Read the model definition and answer for the solid it produces. Units are mm, in the model's axes. A direction names the side the tool comes from. Give positions to 0.01 mm unless a question says otherwise; leave off trailing zeros. Order: outer loops, then holes, each group sorted by start corner. A loop starts at its lowest first (then second) coordinate and runs counter-clockwise, first axis right, second up. Notation, with made-up numbers: (26.25, 17) -> (36.25, 17) arc R4 cw to (36.25, 23) -> close; hole circle Ø11 at (63, 75.25). An arc over 180 degrees is marked (long way). Answer as CSV lines item,"result". Start each with the question number.
1) Find section D-D (x = 0.75). Determine the outline of the cut face in (y, z), and give its area (3 significant figures).
2) For faces 5 (the face through (0, 15, 6)), 6 (the face through (0, 8.019, 7)), 7 (the face through (-12.5, 4, 5)), determine the directions among +Z, -Z, +X, -X, +Y, -Y from which every point of the face is accessible in a straight line to the end or side of a thin tool.
3) Find section B-B (x = -8.5). Determine the outline of the cut face in (y, z).
4) Find section A-A (y = 2.75). Determine the outline of the cut face in (x, z).
5) Flat-ended cylindrical pins translate along their axes: pin 1 Ø5 at (x, z) = (-9, 3) entering from +Y; pin 2 Ø5 at (y, z) = (19, 5.5) entering from +X; pin 3 Ø3.5 at (x, y) = (0, 17) entering from +Z. Find the tip coordinate at first contact, or state that the pin passes through.
6) Straight lines are drawn through the part: L1, parallel to X at y = 3.5, z = 6.75; L2, parallel to X at y = 2.5, z = 6.5; L3, parallel to Y at x = 11, z = 1. For each, find the intervals that lie inside material, in ascending order. Write a range as from..to.
7) The mould has two halves that part along Y. Classify faces 1 (the face through (7.3, 5.8, 4.9)), 2 (the face through (4.213, 14.921, 2.958)), 3 (the face through (0, 4, 10)), 4 (the face through (-6.478, 5.503, 4.93)): +Y half, -Y half, draft (parallel to the pull), parting line (faces both ways), or undercut.
8) Find section C-C (z = 2). Determine the outline of the cut face in (x, y), and give its area (3 significant figures).
```python
from build123d import *

# Parameters (mm, degrees)
SKETCH001_R  = 2
PAD_DEPTH    = 6
SKETCH_W     = 25
SKETCH_H     = 8.532326
SKETCH_R     = 2
PAD001_DEPTH = 4


with BuildPart() as part:
    # Sketch001 → Pad (new body)
    with BuildSketch(Plane.XY):
        with BuildLine():
            Line((0, -0.513451), (12.5, -0.513451))
            Line((12.5, -0.513451), (12.5, 8.018875))
            Line((12.5, 8.018875), (5.444822, 8.018875))
            Line((5.444822, 8.018875), (2.947073, 22.018734))
            ThreePointArc((2.947073, 22.018734), (1.921936, 23.788122), (0, 24.486549))
            ThreePointArc((0, 24.486549), (-1.921936, 23.788122), (-2.947073, 22.018734))
            Line((-5.444822, 8.018875), (-2.947073, 22.018734))
            Line((-12.5, 8.018875), (-5.444822, 8.018875))
            Line((-12.5, -0.513451), (-12.5, 8.018875))
            Line((0, -0.513451), (-12.5, -0.513451))
        make_face()
        with Locations((-7.553649, 3.816244)):
            Circle(SKETCH001_R, mode=Mode.SUBTRACT)
        with Locations((7.553649, 3.816244)):
            Circle(SKETCH001_R, mode=Mode.SUBTRACT)
    extrude(amount=PAD_DEPTH)

    # Sketch → Pad001 (new body)
    with BuildSketch(Plane.XY.offset(6)):
        with Locations((0, 3.752712)):
            Rectangle(SKETCH_W, SKETCH_H)
        with Locations((-7.553649, 3.816244)):
            Circle(SKETCH_R, mode=Mode.SUBTRACT)
        with Locations((7.553649, 3.816244)):
            Circle(SKETCH_R, mode=Mode.SUBTRACT)
    extrude(amount=PAD001_DEPTH)


solid = part.part
```
Findings below:
1,outline,"(-0.51, 0) -> (24.39, 0) -> (24.39, 6) -> (8.02, 6) -> (8.02, 10) -> (-0.51, 10) -> close"
1,area,"184 mm²"
2,face 5,"+Z, +X, -X, +Y"
2,face 6,"+Z, +Y"
2,face 7,"+Z, -Z, -X, +Y, -Y"
3,outline,"(-0.51, 0) -> (2.05, 0) -> (2.05, 10) -> (-0.51, 10) -> close; (5.58, 0) -> (8.02, 0) -> (8.02, 10) -> (5.58, 10) -> close"
4,outline,"(-12.5, 0) -> (-9.25, 0) -> (-9.25, 10) -> (-12.5, 10) -> close; (-5.86, 0) -> (5.86, 0) -> (5.86, 10) -> (-5.86, 10) -> close; (9.25, 0) -> (12.5, 0) -> (12.5, 10) -> (9.25, 10) -> close"
5,pin 1,"y = 8.02"
5,pin 2,"x = 3.93"
5,pin 3,"z = 6"
6,L1,"-12.5..-9.53, -5.58..5.58, 9.53..12.5"
6,L2,"-12.5..-9.06, -6.05..6.05, 9.06..12.5"
6,L3,"-0.51..8.02"
7,face 1,"undercut"
7,face 2,"+Y half"
7,face 3,"draft"
7,face 4,"undercut"
8,outline,"(-12.5, -0.51) -> (12.5, -0.51) -> (12.5, 8.02) -> (5.44, 8.02) -> (2.95, 22.02) arc R2.99 ccw to (0, 24.49) arc R2.99 ccw to (-2.95, 22.02) -> (-5.44, 8.02) -> (-12.5, 8.02) -> close; hole circle Ø4 at (-7.55, 3.82); hole circle Ø4 at (7.55, 3.82)"
8,area,"317 mm²"
